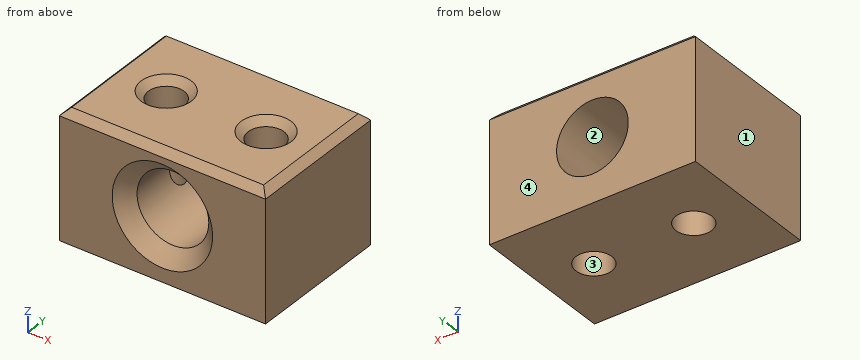
from build123d import *

# Parameters (mm, degrees)
F0_W     = 73.031252
F0_H     = 45.270924
F0_R     = 12.7
F1_DEPTH = 50.8
F3_D     = 12.7
F4_SIZE  = 5.08
F5_SIZE  = 2.54


with BuildPart() as f1:
    # F0 (on Front) → F1 (new body)
    with BuildSketch(Plane.XZ):
        Rectangle(F0_W, F0_H)
        Circle(F0_R, mode=Mode.SUBTRACT)
    extrude(amount=F1_DEPTH)

    # F3 (through all)
    with Locations(Plane.XY.offset(22.635462)):
        with Locations((-17.163437, -25.553048), (18.195821, -25.553048)):
            Hole(F3_D / 2)

    # F4
    f4_edges = [f1.edges().sort_by_distance(p)[0] for p in [
        (-12.7, -50.8, 0),
    ]]
    chamfer(f4_edges, length=F4_SIZE)

    # F5
    f5_edges = [f1.edges().sort_by_distance(p)[0] for p in [
        (36.515626, -25.4, 22.635462),
        (0, 0, 22.635462),
        (0, -50.8, 22.635462),
        (-36.515626, -25.4, 22.635462),
        (11.845821, -25.553048, 22.635462),
        (-23.513437, -25.553048, 22.635462),
    ]]
    chamfer(f5_edges, length=F5_SIZE)


solid = f1.part
Build history of the part. All positions in model axes, mm. Face numbers are marked on the shaded views. Coordinates: 2 decimals unless noted, no trailing zeros. Order: outer loops, then holes, each group sorted by start corner. A loop starts at its lowest first (then second) coordinate and runs counter-clockwise, first axis right, second up. Notation, with made-up numbers: M -37,30.5 L 0,30.5 A12 cw 0,37.5 Z; hole C -22,51.5 d10. An arc over 180 degrees is marked long. One line per question, with ' | ' between items. Start each with the question number.
Q1. Probe L1, parallel to Z at x = 0, y = -12; L2, parallel to X at y = -28, z = 19.5; L3, parallel to X at y = -29, z = -18.5. List the from-to ranges inside material, lowest first. Write a range as from..to.
Q2. Saw through at C-C (y = -43.5). List the corners of the cut face in (x, z), then the cut area to 3 significant figures.
Q3. Saw through at B-B (z = 0). List the corners of the cut face in (x, y), then the cut area to 3 significant figures.
Q4. Two-plate mould, pull along X, no slides. Class the marked faces 1, 2, 3 and 4: +X half, -X half, draft (parallel to the pull), parting line (faces both ways), or undercut.
Q5. Flat gauge pin, fed straight in: pin 1 Ø11.5 at (x, y) = (18.2, -25.55) entering from +Z. Where does the tip first touch, or does it go through?
Q6. Saw through at D-D (z = -6). Count the separate pieces of the cut face and the enclosed holes in it, then the cut area to 3 significant figures.
Q7. Saw through at A-A (x = 0). List the corners of the cut face in (y, z), then the cut area to 3 significant figures.
Check values:
1) L1: z = -22.64..-12.7, 12.7..22.64 | L2: x = -36.52..-23.02, -11.3..12.34, 24.06..36.52 | L3: x = -36.52..-22.5, -11.83..12.86, 23.53..36.52
2) outline: M -36.52,-22.64 L 36.52,-22.64 L 36.52,20.1 L 33.98,22.64 L -33.98,22.64 L -36.52,20.1 Z; hole C 0,0 d25.4 | area: 2,790 mm2
3) outline: M -36.52,-50.8 L -17.78,-50.8 L -12.7,-45.72 L -12.7,-30.07 A6.35 cw long -12.7,-21.04 L -12.7,0 L -36.52,0 Z; M 12.7,-45.72 L 17.78,-50.8 L 36.52,-50.8 L 36.52,0 L 12.7,0 L 12.7,-22.37 A6.35 cw long 12.7,-28.73 Z | area: 2,160 mm2
4) face 1: -X half | face 2: undercut | face 3: undercut | face 4: draft
5) pin 1: passes through
6) separate pieces: 2 | enclosed holes: 1 | area: 2,290 mm2
7) outline: M -50.8,-22.64 L 0,-22.64 L 0,-12.7 L -45.72,-12.7 L -50.8,-17.78 Z; M -50.8,17.78 L -45.72,12.7 L 0,12.7 L 0,20.1 L -2.54,22.64 L -48.26,22.64 L -50.8,20.1 Z | area: 977 mm2
